Read the model definition and answer for the solid it produces. Units are mm, in the model's axes. Round coordinates to 2 decimals unless told otherwise and drop trailing zeros. Order: outer loops, then holes, each group sorted by start corner. A loop starts at its lowest first (then second) coordinate and runs counter-clockwise, first axis right, second up. Notation, with made-up numbers: (9.25, 27) - (13.25, 27) arc R19 cw to (13.25, 38) - close; hole circle Ø8 at (-31.75, -22). An arc over 180 degrees is marked (long way). One line per question, with ' | ' between items. Start each with the question number.
1) The part is cut by section A-A, the plane y = 119.5. Give the vertices of the cut face in (x, z), plus the area to 3 significant figures.
2) The part is cut by section C-C, the plane z = 25. Give the vertices of the cut face in (x, y), plus the area to 3 significant figures.
3) Straight lines are drawn through the part: line 1 (Z direction, x = -77, y = 82); line 2 (Y direction, x = -56, z = 22); line 3 (X direction, y = -98, z = 8). For each, find the intervals that lie inside material, in ascending order. Write a range as from..to.
4) The part is cut by section D-D, the plane y = -48. Give the vertices of the cut face in (x, z), plus the area to 3 significant figures.
5) Flat-ended cylindrical pins translate along their axes: pin 1 (2 mm diameter, centred on x = 94.5, y = 10, fed in from +Z); pin 2 (1.9 mm diameter, centred on y = 64.5, z = 8, fed in from -X); pin 3 (12.5 mm diameter, centred on y = -27, z = 31.5, fed in from +X). Find the tip coordinate at first contact, or state that the pin passes through.
from build123d import *

# Parameters (mm, degrees)
F0_W     = 304.8
F0_H     = 304.8
F0_W_2   = 292.1
F0_H_2   = 292.1
F1_DEPTH = 6.35
F2_DEPTH = 12.7
F3_W     = 114.3
F3_H     = 114.3
F4_DEPTH = 25.4


with BuildPart() as f1:
    # F0 (on Top) → F1 (new body)
    with BuildSketch(Plane.XY):
        Rectangle(F0_W, F0_H)
        Rectangle(F0_W_2, F0_H_2, mode=Mode.SUBTRACT)
    extrude(amount=F1_DEPTH)

    # F0 (on Top) → F2 (join)
    with BuildSketch(Plane.XY):
        Rectangle(F0_W_2, F0_H_2)
    extrude(amount=F2_DEPTH)

    # F3 (on face) → F4 (join)
    with BuildSketch(Plane.XY.offset(12.7)):
        Rectangle(F3_W, F3_H)
    extrude(amount=F4_DEPTH)


solid = f1.part
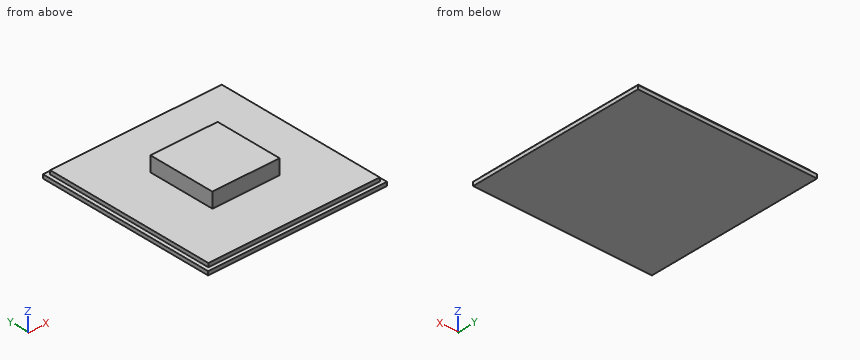
Values:
1) outline: (-152.4, 0) - (152.4, 0) - (152.4, 6.35) - (146.05, 6.35) - (146.05, 12.7) - (-146.05, 12.7) - (-146.05, 6.35) - (-152.4, 6.35) - close | area: 3,790 mm^2
2) outline: (-57.15, -57.15) - (57.15, -57.15) - (57.15, 57.15) - (-57.15, 57.15) - close | area: 13,100 mm^2
3) line 1: z = 0..12.7 | line 2: y = -57.15..57.15 | line 3: x = -146.05..146.05
4) outline: (-152.4, 0) - (152.4, 0) - (152.4, 6.35) - (146.05, 6.35) - (146.05, 12.7) - (57.15, 12.7) - (57.15, 38.1) - (-57.15, 38.1) - (-57.15, 12.7) - (-146.05, 12.7) - (-146.05, 6.35) - (-152.4, 6.35) - close | area: 6,690 mm^2
5) pin 1: stops at z = 12.7 | pin 2: stops at x = -146.05 | pin 3: stops at x = 57.15
